Part model, mm, in its own coordinate system. A direction names the side the tool comes from. Give positions to 0.01 mm unless a question says otherwise; leave off trailing zeros. Write each loop counter-clockwise with the first axis right and the second up, starting at its lowest first coordinate (ties: lowest second). Pieces come first, ordered by that corner, then holes. Notation, with made-up numbers: (-9, -14.75) - (19, -14.75) arc R36 ccw to (19, 21.25) - close; hole circle Ø5 at (50.5, 7.25). An arc over 180 degrees is marked (long way). Answer in a Markdown table with one row per item. Add a question column.
1. Which spindle directions (+Z, -Z, +X, -X, +Y, -Y) get a long thin tool onto all of the face, cutting with end or side? Do faces 5 (the cylindrical face through (-21.462, -21.996, 5.07)), 6 (the cylindrical face through (19.932, -3.228, 3.549)). Say none if no direction does.
2. Band-saw the part on C-C on z = 3. State how many separate pieces and enclosed holes the cut face has, plus the area to 3 significant figures.
3. Band-saw the part on B-B on x = -22.5. Write the cut outline in (y, z), plus the area to 3 significant figures.
4. Pull direction Y, two halves, no side cores. Call faces 1 (the flat face through (30, 0, 5)), 2 (the flat face through (0, 30, 5)), 3 (the cylindrical face through (23.538, 18.004, 5.07)), 4 (the conical face through (-17.058, -3.975, 8.266)): released by +Y, released by -Y, zero draft, split by the parting line, or undercut.
5. Probe line 1 along Y through (x, z) = (0, 5.25); line 2 along X through (y, z) = (-15, 1); line 3 along Y through (x, z) = (19, 4). List the from-to ranges inside material, lowest first.
6. Band-saw the part on A-A on y = 0. Write the cut outline in (x, z).
7. Drop flat-ended pins along their axis: pin 1 Ø4 at (x, y) = (0, -17.95) entering from -Z; pin 2 Ø3 at (x, y) = (0, 17.95) entering from -Z; pin 3 Ø4 at (x, y) = (-22.5, -20) entering from +Z; pin 4 Ø3 at (y, z) = (-22.5, 4.5) entering from +X. Give the stop position or say it passes through.
```python
from build123d import *

# Parameters (mm, degrees)
ESQUISSE1_W                         = 60
ESQUISSE1_H                         = 60
BOSS_EXTRU_1_DEPTH                  = 10
DIAM_TRE_DU_PER_AGE_4_5_4_5_1_D     = 4.5
DIAM_TRE_DU_PER_AGE_5_1_5_1_1_D     = 5.1
DIAM_TRE_DU_PER_AGE_5_1_5_1_1_DEPTH = 7
DIAM_TRE_DU_PER_AGE_5_1_5_1_1_TIP   = 1.532194579
ESQUISSE9_R                         = 13.4
ENL_V_MAT_EXTRU_2_DEPTH             = 44.588989435
CONG_3_R                            = 15


with BuildPart() as part:
    # Esquisse1 → Boss.-Extru.1 (new body)
    with BuildSketch(Plane(origin=(0, 0, 0), x_dir=(-1, 0, 0), z_dir=(0, 0, -1))):
        Rectangle(ESQUISSE1_W, ESQUISSE1_H)
    extrude(amount=-BOSS_EXTRU_1_DEPTH)

    # Diamètre du perçage Ø4.5 (4.5)1 (through all)
    with Locations(Plane(origin=(0, 0, 0), x_dir=(-1, 0, 0), z_dir=(0, 0, -1))):
        with Locations((22.5, 20), (-22.5, 20), (-22.5, -20), (22.5, -20)):
            Hole(DIAM_TRE_DU_PER_AGE_4_5_4_5_1_D / 2)

    # Diamètre du perçage Ø5.1 (5.1)1
    with Locations(Plane(origin=(0, 0, 0), x_dir=(-1, 0, 0), z_dir=(0, 0, -1))):
        with Locations((-14.03387511, 11.191641943), (-7.788213117, 16.172391179), (0, 17.95), (7.788213117, 16.172391179), (14.03387511, 11.191641943), (17.499956024, 3.994250765), (17.499956024, -3.994250765), (14.03387511, -11.191641943), (7.788213117, -16.172391179), (0, -17.95), (-7.788213117, -16.172391179), (-14.03387511, -11.191641943), (-17.499956024, -3.994250765), (-17.499956024, 3.994250765)):
            Hole(DIAM_TRE_DU_PER_AGE_5_1_5_1_1_D / 2, depth=DIAM_TRE_DU_PER_AGE_5_1_5_1_1_DEPTH)
            with Locations((0, 0, -(DIAM_TRE_DU_PER_AGE_5_1_5_1_1_DEPTH + DIAM_TRE_DU_PER_AGE_5_1_5_1_1_TIP / 2))):  # 118° drill point
                Cone(0, DIAM_TRE_DU_PER_AGE_5_1_5_1_1_D / 2, DIAM_TRE_DU_PER_AGE_5_1_5_1_1_TIP, mode=Mode.SUBTRACT)

    # Esquisse9 → Enlèv. mat.-Extru.2 (cut, through all)
    with BuildSketch(Plane(origin=(0, 0, 0), x_dir=(-1, 0, 0), z_dir=(0, 0, -1))):
        Circle(ESQUISSE9_R)
    extrude(amount=-ENL_V_MAT_EXTRU_2_DEPTH, mode=Mode.SUBTRACT)

    # Congé3
    cong_3_edges = [part.edges().sort_by_distance(p)[0] for p in [
        (30, 30, 5),
        (-30, 30, 5),
        (-30, -30, 5),
        (30, -30, 5),
    ]]
    fillet(cong_3_edges, radius=CONG_3_R)


solid = part.part
```
Values:
| question | item | result |
|---|---|---|
| 1 | face 5 | +Z, -Z |
| 1 | face 6 | -Z |
| 2 | separate pieces | 1 |
| 2 | enclosed holes | 19 |
| 2 | area | 2,490 mm² |
| 3 | outline | (-27.99, 0) - (-22.25, 0) - (-22.25, 10) - (-27.99, 10) - close; (-17.75, 0) - (17.75, 0) - (17.75, 10) - (-17.75, 10) - close; (22.25, 0) - (27.99, 0) - (27.99, 10) - (22.25, 10) - close |
| 3 | area | 470 mm² |
| 4 | face 1 | zero draft |
| 4 | face 2 | released by +Y |
| 4 | face 3 | undercut |
| 4 | face 4 | undercut |
| 5 | line 1 | y = -30 to -20.5, -15.4 to -13.4, 13.4 to 15.4, 20.5 to 30 |
| 5 | line 2 | x = -30 to -10.05, -5.52 to 5.52, 10.05 to 30 |
| 5 | line 3 | y = -29.46 to -6.06, -1.93 to 1.93, 6.06 to 29.46 |
| 6 | outline | (-30, 0) - (-13.4, 0) - (-13.4, 10) - (-30, 10) - close; (13.4, 0) - (30, 0) - (30, 10) - (13.4, 10) - close |
| 7 | pin 1 | stops at z = 7.33 |
| 7 | pin 2 | stops at z = 7.63 |
| 7 | pin 3 | passes through |
| 7 | pin 4 | stops at x = 28.75 |
